Check sheet for the modelled part. Datum: model origin and axes. Units: mm. Face numbers are marked on the shaded views. A direction names the side the tool comes from. Give positions to 0.01 mm unless a question says otherwise; leave off trailing zeros. Loops run counter-clockwise (first coordinate to the right, second up) from the corner with the lowest first, then second, coordinate; pieces in that order, holes last. Notation, with made-up numbers: (1, 39.25) - (33, 39.25) arc R9 ccw to (33, 47.25) - close; hole circle Ø3 at (6.5, -1.5). An arc over 180 degrees is marked (long way). Answer in a Markdown table with one row per item. Add a question column.
(1) Sectioned sample at A-A on x = 0. Enter the section's corners in (y, z).
(2) Sectioned sample at C-C on y = -1.5. Enter the section's corners in (x, z).
(3) Go/stop test with a flat-tipped pin: P1, Ø1.5, axis at x = 4, z = -2, coming from the +Y side. Record where the tip stops, or that it passes through.
(4) Sectioned sample at D-D on x = -2.25. Enter the section's corners in (y, z), then the cut area to 3 significant figures.
(5) Set-up check for the marked faces 1, 2 and 3: record each of +Z, -Z, +X, -X, +Y, -Y from which the full face is reachable in a straight line by a thin tool's end or side.
(6) Sectioned sample at B-B on z = 4.5. Enter the section's corners in (x, y).
(7) Thickness scan on L1, parallel to Y at x = 0, z = 4.95; L2, parallel to Z at x = -2, y = -6.75; L3, parallel to Y at x = 0, z = -3. Record the ranges inside material, lowest first.
(8) Draft check along Z on the marked faces 4, 5 and 6. Enter one of: released by +Z, released by -Z, zero draft, split by the parting line, or undercut.
from build123d import *

# Parameters (mm, degrees)
SALIENTE_EXTRUIR1_DEPTH = 5
CROQUIS2_R              = 2
CROQUIS2_R_2            = 2.5
CORTAR_EXTRUIR1_DEPTH   = 12
REDONDEO1_R             = 4


with BuildPart() as part:
    # Croquis1 → Saliente-Extruir1 (new body, symmetric)
    with BuildSketch(Plane(origin=(0, 0, 0), x_dir=(0, 0, -1), z_dir=(1, 0, 0))):
        Polygon((4, 9), (6, 9), (6, -9), (4, -9), (4, -0.5), (-4, -0.5), (-4, -9), (-6, -9), (-6, 9), (-4, 9), (-4, 2), (4, 2), align=None)
    extrude(amount=SALIENTE_EXTRUIR1_DEPTH, both=True)

    # Croquis2 → Cortar-Extruir1 (cut)
    with BuildSketch(Plane(origin=(0, 0, -6), x_dir=(-1, 0, 0), z_dir=(0, 0, -1))):
        with Locations((0, 6)):
            Circle(CROQUIS2_R)
        with Locations((0, -5)):
            Circle(CROQUIS2_R_2)
    extrude(amount=-CORTAR_EXTRUIR1_DEPTH, mode=Mode.SUBTRACT)

    # Redondeo1
    redondeo1_edges = [part.edges().sort_by_distance(p)[0] for p in [
        (-5, -9, -5),
        (-5, -9, 5),
        (-5, 9, 5),
        (-5, 9, -5),
        (5, 9, 5),
        (5, -9, 5),
        (5, -9, -5),
        (5, 9, -5),
    ]]
    fillet(redondeo1_edges, radius=REDONDEO1_R)


solid = part.part
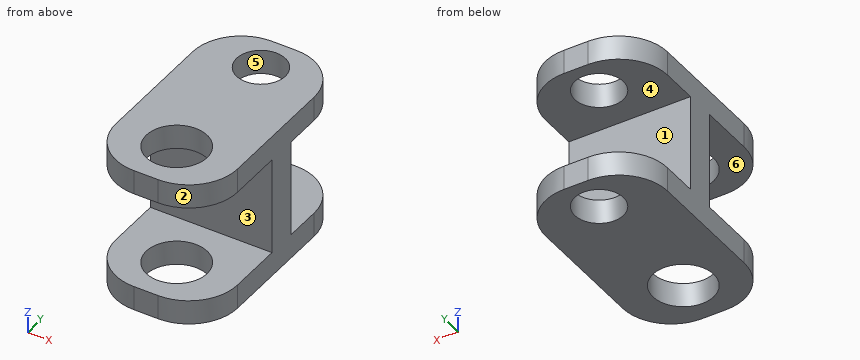
Reply:
| question | item | result |
|---|---|---|
| 1 | outline | (-9, -6) - (-7.5, -6) - (-7.5, -4) - (-9, -4) - close; (-9, 4) - (-7.5, 4) - (-7.5, 6) - (-9, 6) - close; (-2.5, -6) - (4, -6) - (4, -4) - (2, -4) - (2, 4) - (4, 4) - (4, 6) - (-2.5, 6) - (-2.5, 4) - (-0.5, 4) - (-0.5, -4) - (-2.5, -4) - close; (8, -6) - (9, -6) - (9, -4) - (8, -4) - close; (8, 4) - (9, 4) - (9, 6) - (8, 6) - close |
| 2 | outline | (-5, -6) - (5, -6) - (5, -4) - (-5, -4) - close; (-5, 4) - (5, 4) - (5, 6) - (-5, 6) - close |
| 3 | P1 | y = 2 |
| 4 | outline | (-8.8, -6) - (-6.09, -6) - (-6.09, -4) - (-8.8, -4) - close; (-8.8, 4) - (-6.09, 4) - (-6.09, 6) - (-8.8, 6) - close; (-3.91, -6) - (8.8, -6) - (8.8, -4) - (2, -4) - (2, 4) - (8.8, 4) - (8.8, 6) - (-3.91, 6) - (-3.91, 4) - (-0.5, 4) - (-0.5, -4) - (-3.91, -4) - close |
| 4 | area | 81.7 mm^2 |
| 5 | face 1 | +X, -X, +Y |
| 5 | face 2 | +Z, -Z, +X, -Y |
| 5 | face 3 | +X, -X, -Y |
| 6 | outline | (-5, -5) arc R4 ccw to (-1, -9) - (1, -9) arc R4 ccw to (5, -5) - (5, 5) arc R4 ccw to (1, 9) - (-1, 9) arc R4 ccw to (-5, 5) - close; hole circle Ø5 at (0, -5); hole circle Ø4 at (0, 6) |
| 7 | L1 | -9 to -7.5, -2.5 to 4, 8 to 9 |
| 7 | L2 | -6 to -4, 4 to 6 |
| 7 | L3 | -0.5 to 2 |
| 8 | face 4 | undercut |
| 8 | face 5 | zero draft |
| 8 | face 6 | undercut |
